Read the model definition and answer for the solid it produces. Units are mm, in the model's axes. Coordinates: 2 decimals unless noted, no trailing zeros. Loops run counter-clockwise (first coordinate to the right, second up) from the corner with the lowest first, then second, coordinate; pieces in that order, holes last.
from build123d import *

# Parameters (mm, degrees)
SKETCH1_R           = 2.5
BOSS_EXTRUDE1_DEPTH = 1


with BuildPart() as part:
    # Sketch1 → Boss-Extrude1 (new body)
    with BuildSketch(Plane(origin=(0, 0, 0), x_dir=(1, 0, 0), z_dir=(0, 1, 0))):
        Polygon((0, 0), (0, 5), (-30, 5), (-30, 143), (0, 143), (0, 148), (5, 148), (5, 178), (295, 178), (295, 148), (300, 148), (300, 143), (330, 143), (330, 5), (300, 5), (300, 0), (295, 0), (295, -30), (5, -30), (5, 0), align=None)
        with Locations(Location((20, -20, 0), (0, 0, 270))):
            Circle(SKETCH1_R, mode=Mode.SUBTRACT)
        with Locations(Location((60, -20, 0), (0, 0, 270))):
            Circle(SKETCH1_R, mode=Mode.SUBTRACT)
        with Locations(Location((280, -20, 0), (0, 0, 270))):
            Circle(SKETCH1_R, mode=Mode.SUBTRACT)
        with Locations(Location((240, -20, 0), (0, 0, 270))):
            Circle(SKETCH1_R, mode=Mode.SUBTRACT)
        with Locations(Location((320, 19, 0), (0, 0, 270))):
            Circle(SKETCH1_R, mode=Mode.SUBTRACT)
        with Locations(Location((320, 129, 0), (0, 0, 270))):
            Circle(SKETCH1_R, mode=Mode.SUBTRACT)
        with Locations(Location((280, 168, 0), (0, 0, 270))):
            Circle(SKETCH1_R, mode=Mode.SUBTRACT)
        with Locations(Location((240, 168, 0), (0, 0, 270))):
            Circle(SKETCH1_R, mode=Mode.SUBTRACT)
        with Locations(Location((60, 168, 0), (0, 0, 270))):
            Circle(SKETCH1_R, mode=Mode.SUBTRACT)
        with Locations(Location((20, 168, 0), (0, 0, 270))):
            Circle(SKETCH1_R, mode=Mode.SUBTRACT)
        with Locations(Location((-20, 129, 0), (0, 0, 270))):
            Circle(SKETCH1_R, mode=Mode.SUBTRACT)
        with Locations(Location((-20, 19, 0), (0, 0, 270))):
            Circle(SKETCH1_R, mode=Mode.SUBTRACT)
        with Locations(Location((-20, 74, 0), (0, 0, 270))):
            Circle(SKETCH1_R, mode=Mode.SUBTRACT)
        with Locations(Location((320, 74, 0), (0, 0, 270))):
            Circle(SKETCH1_R, mode=Mode.SUBTRACT)
    extrude(amount=BOSS_EXTRUDE1_DEPTH)


solid = part.part
Q1. A cutting plane is placed at B-B (z = -156). Give the vertices of the cut face in (x, y).
Findings below:
outline: (5, 0) - (295, 0) - (295, 1) - (5, 1) - close
Q2. Straight lines are drawn through the part: probe 1 along X at (y, z) = (0.3, -168); probe 2 along X at (y, z) = (0.55, -74); probe 3 along X at (y, z) = (0.55, 21.5). For each, find the intervals that lie inside material, in ascending order.
Findings below:
probe 1: x = 5 to 17.5, 22.5 to 57.5, 62.5 to 237.5, 242.5 to 277.5, 282.5 to 295
probe 2: x = -30 to -22.5, -17.5 to 317.5, 322.5 to 330
probe 3: x = 5 to 18, 22 to 58, 62 to 238, 242 to 278, 282 to 295
Q3. Flat-ended cylindrical pins translate along their axes: pin 1 Ø6.5 at (x, z) = (320, -129) entering from -Y; pin 2 Ø0.5 at (y, z) = (0.5, -3) entering from -X; pin 3 Ø0.5 at (x, y) = (2, 0.5) entering from -Z. Find the tip coordinate at first contact, or state that the pin passes through.
Findings below:
pin 1: stops at y = 0
pin 2: stops at x = 0
pin 3: stops at z = -148
Q4. A cutting plane is placed at A-A (y = 0.7). Count the separate pieces of the cut face and the enclosed holes in it, then the cut area to 3 significant figures.
Findings below:
separate pieces: 1
enclosed holes: 14
area: 69,800 mm2
